from build123d import *

# Parameters (mm, degrees)
SKETCH1_R              = 34.671
BOSS_EXTRUDE1_DEPTH    = 9.525
FILLET1_R              = 5.08
F_10_CLEARANCE_HOLE1_D = 5.1054


with BuildPart() as part:
    # Sketch1 → Boss-Extrude1 (new body)
    with BuildSketch(Plane.XY):
        with Locations(Location((0, 0, 0), (0, 0, 180))):
            Circle(SKETCH1_R)
        with BuildLine():
            ThreePointArc((19.058413969, -22.135965238), (29.21, 0), (19.058413969, 22.135965238))
            ThreePointArc((19.058413969, 22.135965238), (11.8745, 20.567237314), (9.641101249, 27.573053271))
            ThreePointArc((9.641101249, 27.573053271), (-14.605, 25.296602045), (-28.699515217, 5.437088034))
            ThreePointArc((-28.699515217, 5.437088034), (-23.749, 0), (-28.699515217, -5.437088034))
            ThreePointArc((-28.699515217, -5.437088034), (-14.605, -25.296602045), (9.641101249, -27.573053271))
            ThreePointArc((9.641101249, -27.573053271), (11.8745, -20.567237314), (19.058413969, -22.135965238))
        make_face(mode=Mode.SUBTRACT)
    extrude(amount=BOSS_EXTRUDE1_DEPTH)

    # Fillet1
    fillet1_edges = [part.edges().sort_by_distance(p)[0] for p in [
        (-28.699515217, 5.437088034, 4.7625),
        (-28.699515217, -5.437088034, 4.7625),
        (9.641101249, -27.573053271, 4.7625),
        (19.058413969, -22.135965238, 4.7625),
        (19.058413969, 22.135965238, 4.7625),
        (9.641101249, 27.573053271, 4.7625),
    ]]
    fillet(fillet1_edges, radius=FILLET1_R)

    # #10 Clearance Hole1 (through all)
    with Locations(Plane(origin=(0, 0, 0), x_dir=(-1, 0, 0), z_dir=(0, 0, -1))):
        with Locations((-14.605, 25.296602045), (29.21, 0), (-14.605, -25.296602045)):
            Hole(F_10_CLEARANCE_HOLE1_D / 2)


solid = part.part
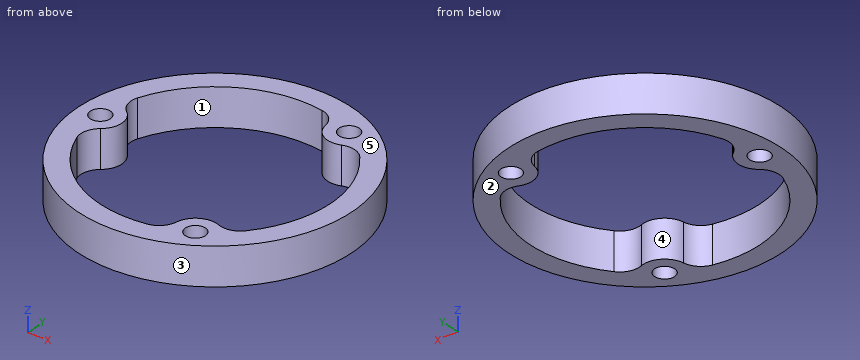
Design review of the part built by this model. Coordinates are the model's own, in mm. Face numbers are marked on the shaded views. A direction names the side the tool comes from. Round coordinates to 2 decimals unless told otherwise and drop trailing zeros. Write each loop counter-clockwise with the first axis right and the second up, starting at its lowest first coordinate (ties: lowest second). Pieces come first, ordered by that corner, then holes.
Item 1: Consider section C-C on x = -29.21. Give the boundary of the cut face in (y, z) (3 decimals).
Item 2: Consider section B-B on x = 0. Give the boundary of the cut face in (y, z) (3 decimals).
Item 3: Consider section A-A on y = 0. Give the boundary of the cut face in (x, z) (3 decimals), and give its area (3 significant figures).
Item 4: Wall thickness on L1, parallel to X at y = -0.5, z = 7.75; L2, parallel to X at y = 26, z = 0.5; L3, parallel to Y at x = 14, z = 0.5: over which ranges is each line inside the solid? List them lowest first.
Item 5: For pin 1 Ø12 at (x, y) = (13.5, -12) entering from -Z; pin 2 Ø6 at (x, y) = (14.6, 25.3) entering from -Z; pin 3 Ø2 at (y, z) = (-11, 1.5) entering from +X; pin 4 Ø1 at (y, z) = (-8.5, 7.5) entering from +X, all flat-tipped, find the tip position at first contact; note any pin that passes through.
Item 6: Draft analysis for pull direction X (two halves, no side actions). For the marked faces 3, 4 and 5, state which applies: released by +X, released by -X, zero draft, split by the parting line, or undercut.
Item 7: Consider section D-D on z = 4.25. Count the separate pieces of the cut face and the enclosed holes in it, and give its area (3 significant figures).
Item 8: For the marked faces 1 and 2, list the 3-axis set-ups (+Z, -Z, +X, -X, +Y, -Y) from which the entire face can be reached by the end or side of a thin tool; tool diameter is ignored.
Check values:
1. outline: (-18.678, 0) - (-2.553, 0) - (-2.553, 9.525) - (-18.678, 9.525) - close; (2.553, 0) - (18.678, 0) - (18.678, 9.525) - (2.553, 9.525) - close
2. outline: (-34.671, 0) - (-29.21, 0) - (-29.21, 9.525) - (-34.671, 9.525) - close; (29.21, 0) - (34.671, 0) - (34.671, 9.525) - (29.21, 9.525) - close
3. outline: (-34.671, 0) - (-31.763, 0) - (-31.763, 9.525) - (-34.671, 9.525) - close; (-26.657, 0) - (-23.749, 0) - (-23.749, 9.525) - (-26.657, 9.525) - close; (29.21, 0) - (34.671, 0) - (34.671, 9.525) - (29.21, 9.525) - close
3. area: 107 mm2
4. L1: x = -34.67 to -31.71, -26.71 to -23.77, 29.21 to 34.67
4. L2: x = -22.94 to -13.31, 8.74 to 12.15, 17.06 to 22.94
4. L3: y = -31.72 to -27.78, -22.82 to -19.87, 19.87 to 22.82, 27.78 to 31.72
5. pin 1: passes through
5. pin 2: stops at z = 0
5. pin 3: stops at x = 33.2
5. pin 4: stops at x = 33.74
6. face 3: split by the parting line
6. face 4: undercut
6. face 5: zero draft
7. separate pieces: 1
7. enclosed holes: 4
7. area: 1,190 mm2
8. face 1: +Z, -Z
8. face 2: -Z, +X, -X, +Y, -Y
